Design review of the part shown in the three views and the two pictorial views. Dimensions are in mm from the part's minimum x, y and z. Round coordinates to 2 decimals unless told otherwise and drop trailing zeros. Loops run counter-clockwise (first coordinate to the right, second up) from the corner with the lowest first, then second, coordinate; pieces in that order, holes last. Notation, with made-up numbers: M -36.75,69 L 1.25,69 A16 ccw 1.25,93 Z; hole C -31.5,57 d9. An arc over 180 degrees is marked long. One line per question, with ' | ' between items.
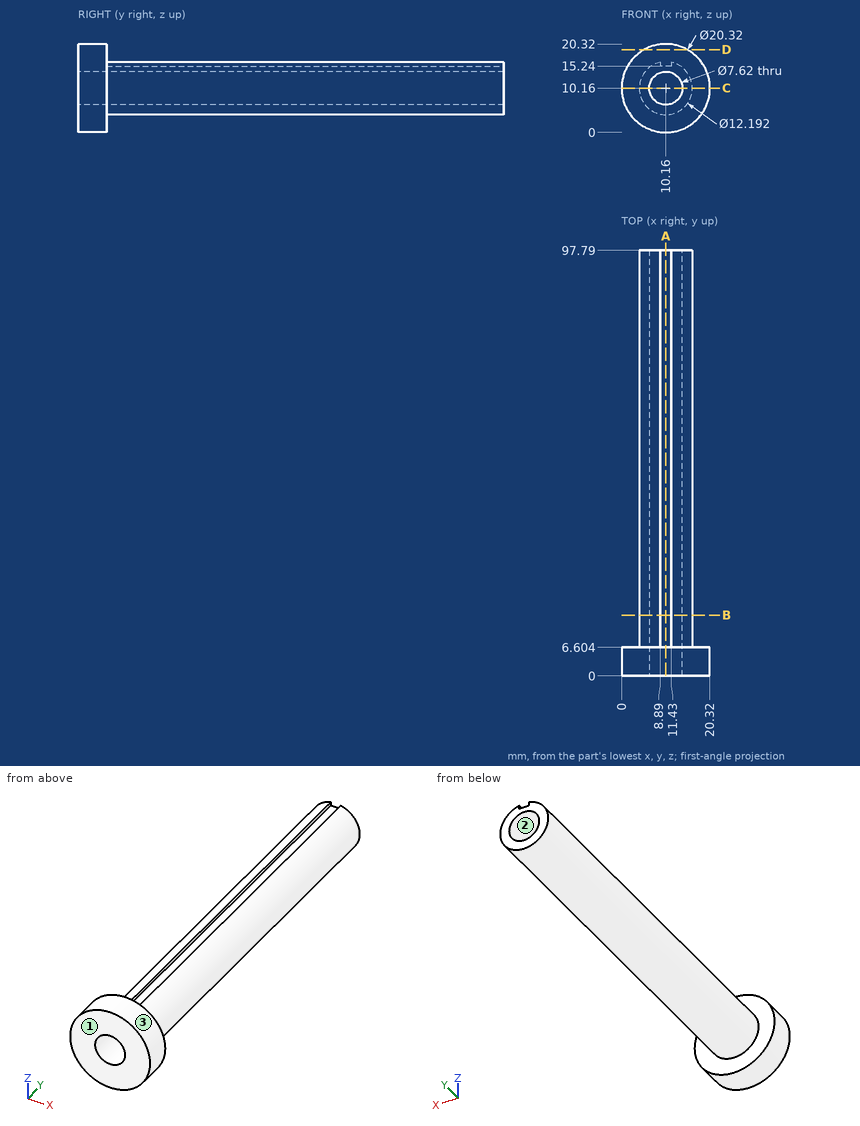
1) Add section C-C on z = 10.16. State the section outline as (x, y) points, then the cut area to 3 significant figures.
Output values:
outline: M 0,0 L 6.35,0 L 6.35,97.79 L 4.06,97.79 L 4.06,6.6 L 0,6.6 Z; M 13.97,0 L 20.32,0 L 20.32,6.6 L 16.26,6.6 L 16.26,97.79 L 13.97,97.79 Z | area: 501 mm²
2) Add section A-A on x = 10.16. State the section outline as (y, z) points.
Output values:
outline: M 0,0 L 6.6,0 L 6.6,4.06 L 97.79,4.06 L 97.79,6.35 L 0,6.35 Z; M 0,13.97 L 97.79,13.97 L 97.79,15.24 L 6.6,15.24 L 6.6,20.32 L 0,20.32 Z
3) Add section D-D on z = 19. State the section outline as (x, y) points.
Output values:
outline: M 5.15,0 L 15.17,0 L 15.17,6.6 L 5.15,6.6 Z
4) For line 1 (X direction, y = 72, z = 10.16); line 2 (Y direction, x = 1.75, z = 15); line 3 (X direction, y = 61, z = 11), list the stretches that pass through material, from the lowest coordinate up.
Output values:
line 1: x = 4.06 to 6.35, 13.97 to 16.26 | line 2: y = 0 to 6.6 | line 3: x = 4.12 to 6.44, 13.88 to 16.2
5) Mouldability with a two-part tool opening along Z and no side actions: class the marked faces 1, 2 and 3 as +Z half, -Z half, draft (parallel to the pull), parting line (faces both ways), or undercut.
Output values:
face 1: draft | face 2: undercut | face 3: parting line
6) Add section B-B on y = 14. State the section outline as (x, z) points, then the cut area to 3 significant figures.
Output values:
outline: M 8.89,15.24 L 8.89,16.12 A6.1 ccw long 11.43,16.12 L 11.43,15.24 Z; hole C 10.16,10.16 d7.62 | area: 68.7 mm²
7) Insertion check: P1, Ø4, axis at x = 16.5, y = 14.5, coming from the -Z side; P2, Ø4.5, axis at x = 10.16, z = 10.16, coming from the +Y side; P3, Ø1.5, axis at x = 15.5, z = 9, coming from the -Y side; P4, Ø1, axis at y = 74, z = 15.5, coming from the +X side. Each pin has a flat end and moves straight along its axis. Give the tip position at first contact, or say it passes through.
Output values:
P1: stops at z = 5.88 | P2: passes through | P3: stops at y = 0 | P4: stops at x = 13.87
